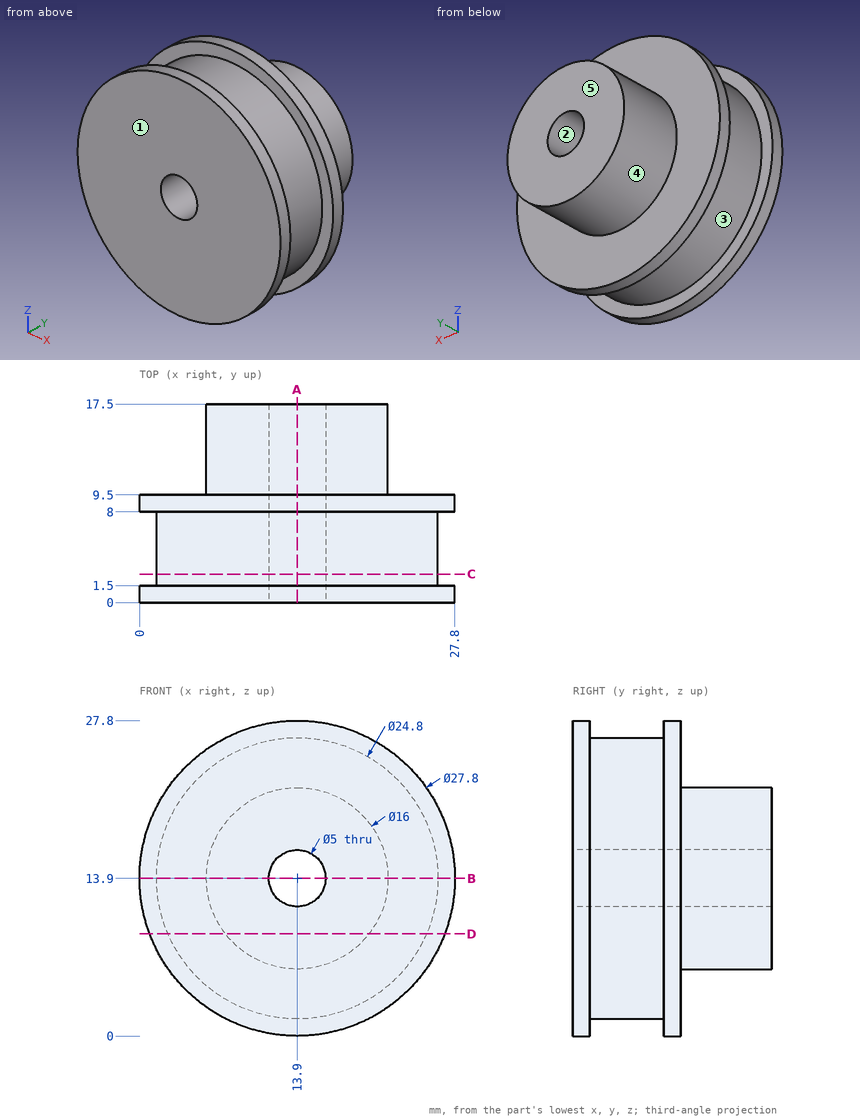
The drawing under review shows one solid part. Ordinate dimensions are in mm from its lowest x, y, z. A direction names the side the tool comes from. Give positions to 0.01 mm unless a question says otherwise; leave off trailing zeros. Loops run counter-clockwise (first coordinate to the right, second up) from the corner with the lowest first, then second, coordinate; pieces in that order, holes last. Notation, with made-up numbers: M -11,-16 L 33,-16 A30 ccw 33,23 Z; hole C -37.75,9 d3. An arc over 180 degrees is marked long. One line per question, with ' | ' between items. Start each with the question number.
1. Add section B-B (z = 13.9). Write out the cut boundary in (x, y), plus the area to 3 significant figures.
2. The part is to be moulded in two halves that separate along Z. For the marked faces 1, 2 and 3, say which applies: released by +Z, released by -Z, zero draft, split by the parting line, or undercut.
3. For the marked faces 4 and 5, list the 3-axis set-ups (+Z, -Z, +X, -X, +Y, -Y) from which the entire face can be reached by the end or side of a thin tool; tool diameter is ignored.
4. Insertion check: P1, Ø10, axis at x = 6.5, y = 15, coming from the +Z side; P2, Ø1, axis at x = 18, y = 11.5, coming from the -Z side; P3, Ø1, axis at y = 9, z = 15, coming from the +X side. Each pin has a flat end and moves straight along its axis. Give the tip position at first contact, or say it passes through.
5. To check wall thickness, follow L1, parallel to Y at x = 6, z = 25; L2, parallel to Y at x = 20.25, z = 6; L3, parallel to X at y = 6, z = 13.9. State the ranges of each line that lie inside material, in increasing order.
6. Add section D-D (z = 9). Write out the cut boundary in (x, y), plus the area to 3 significant figures.
7. Add section A-A (x = 13.9). Write out the cut boundary in (y, z).
8. Add section C-C (y = 2.5). Write out the cut boundary in (x, z).
Worked out:
1) outline: M 0,0 L 11.4,0 L 11.4,17.5 L 5.9,17.5 L 5.9,9.5 L 0,9.5 L 0,8 L 1.5,8 L 1.5,1.5 L 0,1.5 Z; M 16.4,0 L 27.8,0 L 27.8,1.5 L 26.3,1.5 L 26.3,8 L 27.8,8 L 27.8,9.5 L 21.9,9.5 L 21.9,17.5 L 16.4,17.5 Z | area: 285 mm²
2) face 1: zero draft | face 2: undercut | face 3: split by the parting line
3) face 4: +Y | face 5: +Z, -Z, +X, -X, +Y
4) P1: stops at z = 21.53 | P2: stops at z = 6.76 | P3: stops at x = 27.79
5) L1: y = 0 to 1.5, 8 to 9.5 | L2: y = 0 to 9.5 | L3: x = 1.5 to 11.4, 16.4 to 26.3
6) outline: M 0.89,0 L 26.91,0 L 26.91,1.5 L 25.29,1.5 L 25.29,8 L 26.91,8 L 26.91,9.5 L 20.22,9.5 L 20.22,17.5 L 7.58,17.5 L 7.58,9.5 L 0.89,9.5 L 0.89,8 L 2.51,8 L 2.51,1.5 L 0.89,1.5 Z | area: 327 mm²
7) outline: M 0,0 L 1.5,0 L 1.5,1.5 L 8,1.5 L 8,0 L 9.5,0 L 9.5,5.9 L 17.5,5.9 L 17.5,11.4 L 0,11.4 Z; M 0,16.4 L 17.5,16.4 L 17.5,21.9 L 9.5,21.9 L 9.5,27.8 L 8,27.8 L 8,26.3 L 1.5,26.3 L 1.5,27.8 L 0,27.8 Z
8) outline: C 13.9,13.9 d24.8; hole C 13.9,13.9 d5
